Autodesk Inventor part; units mm, degrees
ref_plane "YZ Plane" through (0, 0, 0) normal (1, 0, 0) x (0, 1, 0)
ref_plane "XZ Plane" through (0, 0, 0) normal (0, 1, 0) x (-1, 0, 0)
ref_plane "XY Plane" through (0, 0, 0) normal (0, 0, 1) x (1, 0, 0)
sketch "Sketch1" plane through (0, 0, 0) normal (0, 0, 1) x (1, 0, 0)
  line L0 (-6.35, -9.861) -> (6.35, -9.861)
  line L1 (6.35, -9.861) -> (6.35, 9.861)
  line L2 (6.35, 9.861) -> (-6.35, 9.861)
  line L3 (-6.35, 9.861) -> (-6.35, -9.861)
  line L4 (-6.35, -9.861) -> (6.35, 9.861) construction
  line L5 (6.35, -9.861) -> (-6.35, 9.861) construction
  point P0 (0, 0)
  dimension "d0" = 12.7
extrude "Extrusion1" add sketch "Sketch1" along normal blind 6.35
fillet "Fillet1" radius 1.5875 9 edges at (6.35, 0, 6.35) (6.35, 9.861, 3.175) (0, 9.861, 6.35) (0, 9.861, 0) (6.35, 0, 0) (0, -9.861, 6.35) (0, -9.861, 0) (-6.35, 0, 0) (-6.35, 0, 6.35)
properties part number "Motor Controller"
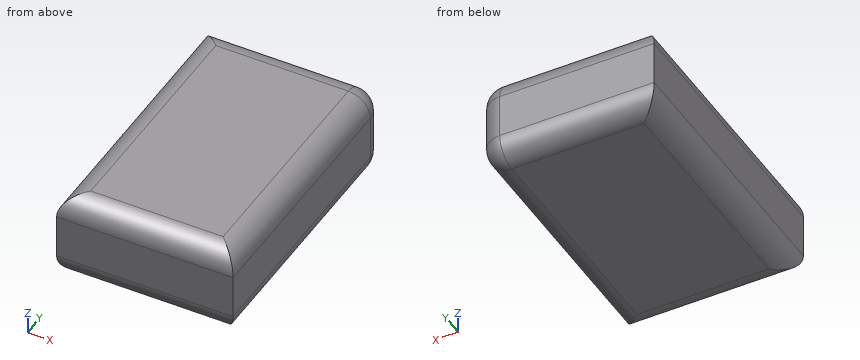
Verification items for the finished model (mm, model axes). Round coordinates to 2 decimals unless told otherwise and drop trailing zeros. Loops run counter-clockwise (first coordinate to the right, second up) from the corner with the lowest first, then second, coordinate; pieces in that order, holes last. Notation, with made-up numbers: (78, 75) - (117, 75) arc R23 cw to (117, 87) - close; hole circle Ø8 at (60, 16.25). An arc over 180 degrees is marked (long way). Answer in a Markdown table with one row per item. Add a question column.
Q1. Material ranges on line 1 (X direction, y = -4.5, z = 1.5); line 2 (Z direction, x = 0, y = 9); line 3 (Y direction, x = 1, z = 6), recorded low to high.
Q2. Section check D-D on z = 0.5. Enter the section's corners in (x, y), plus the area to 3 significant figures.
Q3. Gauge pin test, flat end, axial feed: pin 1 (1.5 mm diameter, centred on y = 1.5, z = 1, fed in from -X). Record the tip position at first contact, or that the pin passes through.
Q4. Section check C-C on z = 6. Enter the section's corners in (x, y), plus the area to 3 significant figures.
Found:
| question | item | result |
|---|---|---|
| 1 | line 1 | x = -6.35 to 6.35 |
| 1 | line 2 | z = 0.18 to 6.17 |
| 1 | line 3 | y = -9.27 to 9.27 |
| 2 | outline | (-5.92, -9.43) - (5.92, -9.43) - (5.92, 8.27) arc R1.16 ccw to (4.76, 9.43) - (-5.92, 9.43) - close |
| 2 | area | 223 mm² |
| 3 | pin 1 | stops at x = -6.35 |
| 4 | outline | (-5.76, -9.27) - (5.76, -9.27) - (5.76, 8.27) arc R0.99 ccw to (4.76, 9.27) - (-5.76, 9.27) - close |
| 4 | area | 213 mm² |
